Source: CAD feature listing. Evaluate the final solid. Frame: model axes, mm. Face numbers are marked on the shaded views. A direction names the side the tool comes from. Give positions to 0.01 mm unless a question says otherwise; leave off trailing zeros. Loops run counter-clockwise (first coordinate to the right, second up) from the corner with the lowest first, then second, coordinate; pieces in that order, holes last. Notation, with made-up numbers: M 83.5,52.25 L 123.5,52.25 A22 ccw 123.5,86.25 Z; hole C 19,20 d6. An arc over 180 degrees is marked long. Put each result on its own line as item: value.
Autodesk Inventor part; units mm, degrees
ref_plane "MSC_PF1" through (0, 0, 0) normal (0, 1, 0) x (-1, 0, 0)
ref_plane "MSC_PT1" through (0, 0, 4.4769) normal (0, 0, -1) x (-1, 0, 0)
ref_plane "YZ Plane" through (0, 0, 0) normal (1, 0, 0) x (0, 1, 0)
sketch "Sketch2" plane through (0, 0, 0) normal (0, 1, 0) x (-1, 0, 0)
  line L0 (0, 4.4769) -> (0, -40.5231)
  line L1 (0, -40.5231) -> (5.125, -40.5231)
  line L2 (6, -39.6481) -> (6, -10.5231)
  line L3 (6, -10.5231) -> (5.35, -9.3972)
  line L4 (5.35, -9.3972) -> (5.35, 4.4769)
  line L5 (5.35, 4.4769) -> (0, 4.4769)
  line L6 (5.125, -40.5231) -> (6, -39.6481)
  line L7 (6, -40.5231) -> (6, -41.7605)
  line L8 (0, -51.008) -> (0, 13.7244)
  dimension "Ds" = 10.7
  dimension "NND" = 12
  dimension "b" = 30
  dimension "d3" = 30
  dimension "d5" = 45
  dimension "PTC" = 1.75
  dimension "NLG" = 45
revolve "Revolution1" add sketch "Sketch2" angle 360 about axis through (0, 0, 4.4769) along (0, 0, -1)
sketch "Sketch3" plane through (0, 0, 4.4769) normal (0, 0, 1) x (1, 0, 0)
  circle A0 centre (0, 0) radius 5.35
  line L0 (0, 9) -> (5.1962, 9)
  line L1 (5.1962, 9) -> (10.3923, 0)
  line L2 (10.3923, 0) -> (0, 0)
  line L3 (0, 0) -> (0, 9)
  line L4 (0, 9) -> (-5.1962, 9)
  line L5 (-5.1962, 9) -> (-10.3923, 0)
  line L6 (0, -9) -> (5.1962, -9)
  line L7 (5.1962, -9) -> (10.3923, 0)
  line L8 (-5.1962, -9) -> (-10.3923, 0)
  line L9 (0, -9) -> (-5.1962, -9)
  dimension "d9" = 60
  dimension "ParS" = 18
  dimension "msp_d11" = 18
extrude "Extrusion1" add sketch "Sketch3" along normal blind 7.5
sketch "Sketch4" plane through (0, 0, 0) normal (0, 1, 0) x (-1, 0, 0)
  line L0 (-9, 11.9769) -> (-10.3923, 11.9769)
  line L1 (-10.3923, 11.9769) -> (-10.3923, 11.1731)
  line L2 (-10.3923, 11.1731) -> (-9, 11.9769)
  line L3 (0, -0.2242) -> (0, 32.6837)
  line L4 (0, 27.9826) -> (0, 27.1787)
  line L5 (-10.3923, 4.4769) -> (-10.3923, 11.9769)
  line L6 (-5.1962, 11.9769) -> (-10.3923, 11.9769)
  dimension "d14" = 30
  dimension "msp_d15" = 18
revolve "Revolution2" cut sketch "Sketch4" angle 360 about axis through (0, 0, 27.9826) along (0, 0, -1)
sketch "Sketch5" plane through (0, 0, 11.9769) normal (0, 0, 1) x (1, 0, 0)
  arc A0 (7.7942, 4.5) -> (0, 9) centre (0, 0) ccw
  circle A1 centre (0, 0) radius 6.75
  dimension "d27" = 13.5
extrude "Extrusion2" cut sketch "Sketch5" against normal blind 1.5
thread "Thread1"
ref_plane "MSC_PF1" through (0, 0, 0) normal (0, 1, 0) x (-1, 0, 0)
ref_plane "MSC_PT1" through (0, 0, 4.4769) normal (0, 0, -1) x (-1, 0, 0)
fillet "Fillet1" radius 0.6 1 edges at (5.35, 0, 4.4769)
equation "\"msp_d11\" = ParS"
equation "\"msp_d15\" = ParS"
equation "\"d27\" = 0.75 * ParS"
equation "\"d28\" = 0.2 * ParK"
equation "\"d30\" = r"
equation "\"msp_d17\" = b"
equation "\"r\" = 0.6"
equation "\"THREADDIA\" = NND"
properties part number "DIN EN ISO 4015 - M12x45" material "Stainless Steel, 440C"
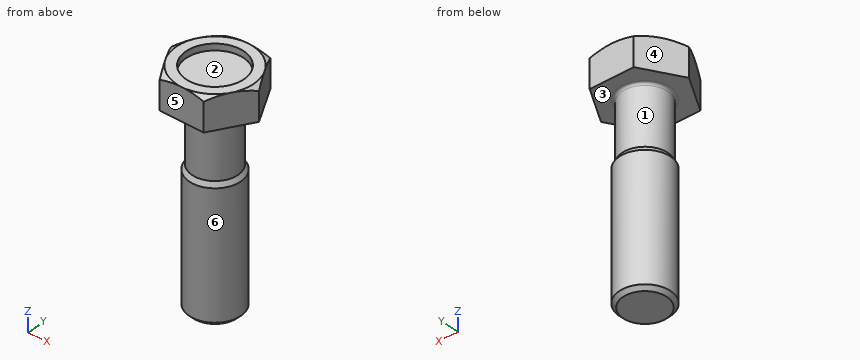
1. Section query B-B (z = -7.5). Output: boundary loops of the cut face in (x, y).
Found:
outline: C 0,0 d10.7
2. Draft query along X for the marked faces 1, 2, 3 and 4. Return one class per face: pulls with the +X half, pulls with the -X half, needs draft (parallel to the pull), parting line crosses it, or undercut.
Found:
face 1: parting line crosses it
face 2: undercut
face 3: needs draft
face 4: pulls with the -X half
3. Section query A-A (z = -24.5). Output: boundary loops of the cut face in (x, y), plus the area to 3 significant figures.
Found:
outline: C 0,0 d12
area: 113 mm^2
4. Material intervals for line 1 (Y direction, x = 0, z = 11.45); line 2 (Z direction, x = 3.75, y = 7); line 3 (X direction, y = 0.25, z = -14), sorted ascending. Write a range as from..to.
Found:
line 1: -9..-6.75, 6.75..9
line 2: 4.48..11.98
line 3: -5.99..5.99
5. Contact query for flat-ended pins moving along their axis: P1, Ø6, axis at y = 5, z = 5.5, coming from the +X side; P2, Ø1, axis at x = 0.5, z = -31.5, coming from the -Y side; P3, Ø1.5, axis at x = 5, y = -0.5, coming from the +Z side; P4, Ø6, axis at x = 5.5, y = 2.5, coming from the -Z side. Output: stop coordinate, or through.
Found:
P1: x = 9.24
P2: y = -6
P3: z = 10.48
P4: z = -40.52
6. Access query for the marked faces 5 and 6. Directions: +Z, -Z, +X, -X, +Y, -Y. A direction counts if a zero-diameter tool reaches every point of the face in a straight line with its end or side. Return the directions, or none.
Found:
face 5: +Z, -Z, +X, -X, -Y
face 6: -Z
